Autodesk Inventor part; units mm, degrees
ref_plane "YZ Plane" through (0, 0, 0) normal (1, 0, 0) x (0, 1, 0)
ref_plane "XZ Plane" through (0, 0, 0) normal (0, 1, 0) x (-1, 0, 0)
ref_plane "XY Plane" through (0, 0, 0) normal (0, 0, 1) x (1, 0, 0)
sketch "Эскиз1" plane through (0, 0, 0) normal (0, 1, 0) x (-1, 0, 0)
  line L0 (0, 0) -> (-35, 0)
  line L1 (-35, 0) -> (-35, 30)
  line L2 (-35, 30) -> (0, 30)
  line L3 (0, 30) -> (0, 0)
  line L4 (-17.5, 25) -> (-17.5, 0)
  line L5 (-17.5, 25) -> (-17.5, 15)
  circle A0 centre (-17.5, 15) radius 10
  dimension "d0" = 35
  dimension "d1" = 30
  dimension "d17" = 10
  dimension "d20" = 15
extrude "Выдавливание1" add sketch "Эскиз1" along normal blind 10
thread "Резьба2"
properties part number "Деталь перемещение по резьбе"
Verification items for the finished model (mm, model axes). Give positions to 0.01 mm unless a question says otherwise; leave off trailing zeros. Write each loop counter-clockwise with the first axis right and the second up, starting at its lowest first coordinate (ties: lowest second). Pieces come first, ordered by that corner, then holes. Notation, with made-up numbers: (17, 18) - (52, 18) arc R33 ccw to (52, 56) - close; hole circle Ø5 at (-20, 16). An arc over 180 degrees is marked (long way). Answer as CSV lines item,"result". Start each with the question number.
1. Sectioned sample at B-B (z = 15). Record the boundary of the cut face in (x, y), then the cut area to 3 significant figures.
2. Sectioned sample at C-C (y = 2.75). Record the boundary of the cut face in (x, z).
3. Draft check along X on faces 1 (the face through (35, 5, 15)), 2 (the face through (17, 5, 0)), 3 (the face through (7.96, 4.93, 12)). Enter one of: pulls with the +X half, pulls with the -X half, needs draft (parallel to the pull), parting line crosses it, or undercut.
4. Thickness scan on line 1 (Z direction, x = 17.5, y = 7.25); line 2 (Z direction, x = 12, y = 7.5); line 3 (X direction, y = 1.5, z = 16.5). Record the ranges inside material, lowest first.
5. Sectioned sample at A-A (x = 17.5). Record the boundary of the cut face in (y, z).
Derived:
1,outline,"(0, 0) - (7.5, 0) - (7.5, 10) - (0, 10) - close; (27.5, 0) - (35, 0) - (35, 10) - (27.5, 10) - close"
1,area,"150 mm²"
2,outline,"(0, 0) - (35, 0) - (35, 30) - (0, 30) - close; hole circle Ø20 at (17.5, 15)"
3,face 1,"pulls with the +X half"
3,face 2,"needs draft"
3,face 3,"undercut"
4,line 1,"0 to 5, 25 to 30"
4,line 2,"0 to 6.65, 23.35 to 30"
4,line 3,"0 to 7.61, 27.39 to 35"
5,outline,"(0, 0) - (10, 0) - (10, 5) - (0, 5) - close; (0, 25) - (10, 25) - (10, 30) - (0, 30) - close"
